Autodesk Inventor part; units mm, degrees
ref_plane "YZ Plane" through (0, 0, 0) normal (1, 0, 0) x (0, 1, 0)
ref_plane "XZ Plane" through (0, 0, 0) normal (0, 1, 0) x (-1, 0, 0)
ref_plane "XY Plane" through (0, 0, 0) normal (0, 0, 1) x (1, 0, 0)
sketch "Sketch2" plane through (0, 0, 0) normal (1, 0, 0) x (0, 1, 0)
  circle A0 centre (0, 0) radius 10
  circle A1 centre (0, 0) radius 22
  line L0 (0, 0) -> (7.0711, -7.0711)
  line L1 (0, 0) -> (10, 0) construction
  circle A2 centre (7.0711, -7.0711) radius 1.5
  line L2 (0, 0) -> (10.8294, 10.8294)
  line L3 (0, 0) -> (15.315, 0) construction
  circle A3 centre (-7.0711, 7.0711) radius 1.5
  dimension "d3" = 20
  dimension "d4" = 44
  dimension "d16" = 10
  dimension "d17" = 45
  dimension "d18" = 3
  dimension "d19" = 45
extrude "Extrusion1" add sketch "Sketch2" along normal blind 12 contours A2 A0 | A0 L0 A2 | A3 A0 | A0 A3 | A0 A2 L0 | A1
sketch "Sketch4" plane through (0, 0, 0) normal (1, 0, 0) x (0, 0, -1)
  circle A0 centre (0, 0) radius 15.75
  circle A1 centre (15.75, 0) radius 2.55
  dimension "d9" = 31.5
  dimension "d10" = 5.1
extrude "Extrusion3" cut sketch "Sketch4" along normal blind 30 contours A0 A1 | A0 A1 picked at (14.9184, -0.4924) picked at (16.4994, -0.6699)
sketch "Sketch5" plane through (12, 0, 0) normal (1, 0, 0) x (0, 0, -1)
  circle A0 centre (15.75, 0) radius 2.55
  circle A1 centre (15.75, 0) radius 4.5
  point P0 (0, 0)
  dimension "d20" = 9
extrude "Extrusion4" cut sketch "Sketch5" against normal blind 6
pattern_circular "Circular Pattern1" count 4 over 360 about axis through (-10, 0, 0) along (1, 0, 0) of "Extrusion3", "Extrusion4"
sketch "Sketch6" plane through (12, 0, 0) normal (1, 0, 0) x (0, 0, -1)
  line L0 (0, 0) -> (15.5563, 15.5563)
  line L1 (0, 0) -> (22, 0) construction
  dimension "d23" = 22
  dimension "d24" = 45
ref_plane "Work Plane1" through (12, 15.5563, -15.5563) normal (0, 0.7071, -0.7071) x (-1, 0, 0)
sketch "Sketch7" plane through (12, 15.5563, -15.5563) normal (0, 0.7071, -0.7071) x (-1, 0, 0)
  line L0 (0, 22) -> (0, -22)
  line L1 (0, 0) -> (12, 0)
  circle A0 centre (6, 0) radius 2.6
  dimension "d25" = 5.2
extrude "Extrusion5" cut sketch "Sketch7" against normal blind 10
ref_plane "Work Plane2" through (12, 0, 0) normal (0, 0.7071, -0.7071) x (-1, 0, 0)
thread "Thread1"
mirror "Mirror1" about plane through (12, 0, 0) normal (0, 0.7071, -0.7071) of "Extrusion5"
properties part number "Pen Holder Interface"
Geometry check sheet. Reference: the model listing, model coordinates, mm. A direction names the side the tool comes from. Give positions to 0.01 mm unless a question says otherwise; leave off trailing zeros. Order: outer loops, then holes, each group sorted by start corner. A loop starts at its lowest first (then second) coordinate and runs counter-clockwise, first axis right, second up. Notation, with made-up numbers: (8.5, -38) - (18.5, -38) arc R10 ccw to (18.5, -19) - close; hole circle Ø10 at (81, -33). An arc over 180 degrees is marked (long way). Use one line per item in the form item = value.
1) Draft check along X on faces 4 (the face through (0, 5, -9)), 5 (the face through (5.96, -8.46, 8.51)), 6 (the face through (6, 2, 18)), 7 (the face through (5.92, 6.93, 7.21)). Enter one of: released by +X, released by -X, zero draft, split by the parting line, or undercut.
Working result:
face_4 = released by -X
face_5 = undercut
face_6 = released by +X
face_7 = zero draft
2) Sectioned sample at B-B (x = 9.75). Record the boundary of the cut face in (y, z).
Working result:
outline = circle Ø44 at (0, 0); hole circle Ø9 at (-15.75, 0); hole (-8.05, 5.93) arc R10 ccw to (5.93, -8.05) arc R1.5 cw to (8.05, -5.93) arc R10 ccw to (-5.93, 8.05) arc R1.5 cw to start; hole circle Ø9 at (0, -15.75); hole circle Ø9 at (0, 15.75); hole circle Ø9 at (15.75, 0)
3) Sectioned sample at A-A (y = 0). Record the boundary of the cut face in (x, z).
Working result:
outline = (0, -22) - (12, -22) - (12, -20.25) - (6, -20.25) - (6, -18.3) - (0, -18.3) - close; (0, -13.2) - (6, -13.2) - (6, -11.25) - (12, -11.25) - (12, -10) - (0, -10) - close; (0, 10) - (12, 10) - (12, 11.25) - (6, 11.25) - (6, 13.2) - (0, 13.2) - close; (0, 18.3) - (6, 18.3) - (6, 20.25) - (12, 20.25) - (12, 22) - (0, 22) - close
4) Sectioned sample at D-D (y = -9). Count the separate pieces of the cut face and the enclosed holes in it, and give its area (3 significant figures).
Working result:
separate_pieces = 2
enclosed_holes = 1
area = 357 mm^2
5) Access from +Z, -Z, +X, -X, +Y, -Y to the whole of each face (thin tool, end or side, straight path). Record for faces 1 (the face through (6, -18, 2)), 2 (the face through (3, -13.2, 0.1)), 3 (the face through (6.04, 8.51, -8.46)).
Working result:
face_1 = +X
face_2 = +X, -X
face_3 = none
6) Depth check by flat-ended pin: pin 1 Ø7 at (y, z) = (-17.5, -2) entering from +X; pin 2 Ø1.5 at (x, y) = (10, -16.5) entering from +Z; pin 3 Ø6 at (x, y) = (5, -5.5) entering from +Z; pin 4 Ø2.5 at (y, z) = (-1.5, 14) entering from +X. Enter the tip coordinate at first touch or a pass-through.
Working result:
pin_1 = 12
pin_2 = 15.36
pin_3 = 21.86
pin_4 = 6
7) Material ranges on probe 1 along Z at (x, y) = (7.75, -12); probe 2 along Z at (x, y) = (11, -2); probe 3 along Y at (x, z) = (6.5, -8.5), recorded low to high. Write a range as from..to.
Working result:
probe_1 = -18.44..-2.49, 2.49..9.28, 14.72..18.44
probe_2 = -21.91..-19.78, -11.72..-9.8, 9.8..11.72, 19.78..21.91
probe_3 = -20.29..-5.27, 5.27..8.47, 12.11..20.29
